Can you work these out from the model? Positions are in its coordinate system, mm. A direction names the side the tool comes from. Give positions to 0.01 mm unless a question says otherwise; leave off trailing zeros. Order: outer loops, then holes, each group sorted by start corner. A loop starts at its lowest first (then second) coordinate and runs counter-clockwise, first axis right, second up. Notation, with made-up numbers: M -40,75 L -25,75 A23 ccw -25,113 Z; hole C 74.25,-10.75 d3. An arc over 180 degrees is marked long. Answer as a JSON object with one key per item and string values.
```python
from build123d import *

# Parameters (mm, degrees)
F1_DEPTH = 17.5
F2_T     = -1.8
F3_R     = 1


with BuildPart() as f1:
    # F0 (on Top) → F1 (new body)
    with BuildSketch(Plane.XY):
        Polygon((-18.35, 10.594377), (-18.35, -10.594377), (0, -21.188755), (18.35, -10.594377), (18.35, 10.594377), (0, 21.188755), align=None)
    extrude(amount=F1_DEPTH)

    # F2
    f2_openings = [f1.faces().sort_by_distance(p)[0] for p in [
        (0, 0, 17.5),
    ]]
    offset(amount=F2_T, openings=f2_openings)

    # F3
    f3_edges = [f1.edges().sort_by_distance(p)[0] for p in [
        (-18.35, 0, 0),
        (-9.175, -15.891566, 0),
        (9.175, -15.891566, 0),
        (18.35, 0, 0),
        (9.175, 15.891566, 0),
        (-9.175, 15.891566, 0),
    ]]
    fillet(f3_edges, radius=F3_R)


solid = f1.part
```
1) I want a section at A-A on z = 15. Write out the boundary of the cut face in (x, y).
Results found:
{"outline": "M -18.35,-10.59 L 0,-21.19 L 18.35,-10.59 L 18.35,10.59 L 0,21.19 L -18.35,10.59 Z; hole M -16.55,-9.56 L 0,-19.11 L 16.55,-9.56 L 16.55,9.56 L 0,19.11 L -16.55,9.56 Z"}
2) For faces 1 (the face through (16.55, 0, 10)), 2 (the face through (0, 0, 0)), which set-ups out of +Z, -Z, +X, -X, +Y, -Y let a thin tool reach every point of the face, with its end or its side?
Results found:
{"face 1": "+Z", "face 2": "-Z, +X, -X, +Y, -Y"}
3) Thinking about a two-plate mould opening in X: for faces 3 (the face through (-8.391, -14.266, 9.54)), 4 (the face through (-9.16, 15.57, 0.3)), 5 (the face through (-16.55, 0, 10)), 6 (the face through (9.16, -15.57, 0.3)), which applies, pulls with the +X half, pulls with the -X half, needs draft (parallel to the pull), parting line crosses it, or undercut?
Results found:
{"face 3": "undercut", "face 4": "pulls with the -X half", "face 5": "undercut", "face 6": "pulls with the +X half"}
4) I want a section at B-B on y = 3. Write out the boundary of the cut face in (x, z).
Results found:
{"outline": "M -18.35,1 A1 ccw -17.35,0 L 17.35,0 A1 ccw 18.35,1 L 18.35,17.5 L 16.55,17.5 L 16.55,1.8 L -16.55,1.8 L -16.55,17.5 L -18.35,17.5 Z"}
5) I'm going to push flat-ended pins straight in: pin 1 Ø5 at (x, z) = (-4, 7.5) entering from -Y; pin 2 Ø1.5 at (y, z) = (-16.5, 15) entering from +X; pin 3 Ø3 at (x, z) = (-10.5, 6.5) entering from -Y. Where does each tip first touch, or does it pass through?
Results found:
{"pin 1": "stops at y = -20.32", "pin 2": "stops at x = 9.42", "pin 3": "stops at y = -15.99"}
6) I need wall thicknesses on L1, parallel to X at y = 1, z = 15.5; L2, parallel to Z at x = 15, y = 0. Which ranges of each line are inside material? Lowest first, please.
Results found:
{"L1": "x = -18.35 to -16.55, 16.55 to 18.35", "L2": "z = 0 to 1.8"}
